The model under review builds one solid part; all positions refer to its coordinate system, in mm. Face numbers are marked on the shaded views. A direction names the side the tool comes from. Give positions to 0.01 mm unless a question says otherwise; leave off trailing zeros. Loops run counter-clockwise (first coordinate to the right, second up) from the corner with the lowest first, then second, coordinate; pieces in that order, holes last. Notation, with made-up numbers: (-2.75, 44) - (23.25, 44) arc R19 cw to (23.25, 50) - close; hole circle Ø8 at (26.5, -32.75). An arc over 180 degrees is marked (long way). Answer as a JSON object with one key per item and string values.
from build123d import *

# Parameters (mm, degrees)
ESQUISSE1_W        = 5
ESQUISSE1_H        = 5
BOSS_EXTRU_1_DEPTH = 5


with BuildPart() as part:
    # Esquisse1 → Boss.-Extru.1 (new body)
    with BuildSketch(Plane.XY):
        with BuildLine():
            Line((-62, 0), (-70, 0))
            Line((-70, 0), (-70, -5))
            Line((-70, -5), (-75, -5))
            Line((-75, -5), (-75, 0))
            Line((-75, 0), (-78.5, 0))
            Line((-78.5, 0), (-78.5, 3))
            Line((-78.5, 3), (-77.4, 3))
            Line((-77.4, 3), (-77.4, 5.3))
            Line((-77.4, 5.3), (-78.5, 5.3))
            Line((-78.5, 5.3), (-78.5, 10))
            Line((-78.5, 10), (-81.5, 10))
            Line((-81.5, 10), (-81.5, 5.3))
            Line((-81.5, 5.3), (-82.6, 5.3))
            Line((-82.6, 5.3), (-82.6, 3))
            Line((-82.6, 3), (-81.5, 3))
            Line((-81.5, 3), (-81.5, 0))
            Line((-81.5, 0), (-85, 0))
            Line((-85, 0), (-85, -5))
            Line((-85, -5), (-90, -5))
            Line((-90, -5), (-90, 0))
            Line((-90, 0), (-98, 0))
            ThreePointArc((-98, 0), (-99.414213562, 0.585786438), (-100, 2))
            Line((-100, 2), (-100, 10))
            Line((-100, 10), (-97.222166499, 42.643036354))
            ThreePointArc((-97.222166499, 42.643036354), (-89.672333618, 59.342381794), (-73.306153302, 67.589578681))
            ThreePointArc((-73.306153302, 67.589578681), (-70.002900284, 68.614551275), (-67.24637377, 70.70347705))
            ThreePointArc((-67.24637377, 70.70347705), (-37.614790527, 91.960082654), (-2.044554135, 99.999503671))
            ThreePointArc((-2.044554135, 99.999503671), (-0.601627423, 99.429879063), (0, 98))
            Line((0, 98), (0, 90))
            Line((0, 90), (5, 90))
            Line((5, 90), (5, 85))
            Line((5, 85), (0, 85))
            Line((0, 85), (0, 81.5))
            Line((0, 81.5), (-3, 81.5))
            Line((-3, 81.5), (-3, 82.6))
            Line((-3, 82.6), (-5.3, 82.6))
            Line((-5.3, 82.6), (-5.3, 81.5))
            Line((-5.3, 81.5), (-10, 81.5))
            Line((-10, 81.5), (-10, 78.5))
            Line((-10, 78.5), (-5.3, 78.5))
            Line((-5.3, 78.5), (-5.3, 77.4))
            Line((-5.3, 77.4), (-3, 77.4))
            Line((-3, 77.4), (-3, 78.5))
            Line((-3, 78.5), (0, 78.5))
            Line((0, 78.5), (0, 75))
            Line((0, 75), (5, 75))
            Line((5, 75), (5, 70))
            Line((5, 70), (0, 70))
            Line((0, 70), (0, 62))
            ThreePointArc((0, 62), (-0.585786438, 60.585786438), (-2, 60))
            Line((-2, 60), (-33.594430088, 60))
            ThreePointArc((-33.594430088, 60), (-41.52653458, 56.08947603), (-43.254902123, 47.416343664))
            ThreePointArc((-43.254902123, 47.416343664), (-42.980213788, 46.295555399), (-42.752787596, 45.164229918))
            ThreePointArc((-42.752787596, 45.164229918), (-43.187469445, 43.527910846), (-44.721399423, 42.811288741))
            Line((-44.721399423, 42.811288741), (-51.993903733, 42.811288741))
            ThreePointArc((-51.993903733, 42.811288741), (-55.195960034, 43.737154782), (-57.409791273, 46.22901026))
            ThreePointArc((-57.409791273, 46.22901026), (-83.571200219, 40.311288741), (-57.409791273, 34.393567223))
            ThreePointArc((-57.409791273, 34.393567223), (-55.195960034, 36.885422701), (-51.993903733, 37.811288741))
            Line((-51.993903733, 37.811288741), (-44.721399423, 37.811288741))
            ThreePointArc((-44.721399423, 37.811288741), (-43.187469445, 37.094666637), (-42.752787596, 35.458347565))
            ThreePointArc((-42.752787596, 35.458347565), (-47.057034679, 24.882654088), (-55.285653392, 16.96674166))
            ThreePointArc((-55.285653392, 16.96674166), (-58.742326175, 13.332888367), (-60, 8.477815449))
            Line((-60, 8.477815449), (-60, 2))
            ThreePointArc((-60, 2), (-60.585786438, 0.585786438), (-62, 0))
        make_face()
        with Locations((-69.821200219, 60.711288741)):
            Rectangle(ESQUISSE1_W, ESQUISSE1_H, mode=Mode.SUBTRACT)
        Polygon((-51.239218472, 53.926352251), (-48.739218472, 49.596225232), (-53.069345491, 47.096225232), (-55.569345491, 51.426352251), align=None, mode=Mode.SUBTRACT)
        Polygon((-48.739218472, 31.026352251), (-51.239218472, 26.696225232), (-55.569345491, 29.196225232), (-53.069345491, 33.526352251), align=None, mode=Mode.SUBTRACT)
        with Locations((-69.821200219, 19.911288741)):
            Rectangle(ESQUISSE1_W, ESQUISSE1_H, mode=Mode.SUBTRACT)
        Polygon((-88.403181966, 26.696225232), (-90.903181966, 31.026352251), (-86.573054947, 33.526352251), (-84.073054947, 29.196225232), align=None, mode=Mode.SUBTRACT)
        Polygon((-90.903181966, 49.596225232), (-88.403181966, 53.926352251), (-84.073054947, 51.426352251), (-86.573054947, 47.096225232), align=None, mode=Mode.SUBTRACT)
    extrude(amount=BOSS_EXTRU_1_DEPTH)


solid = part.part
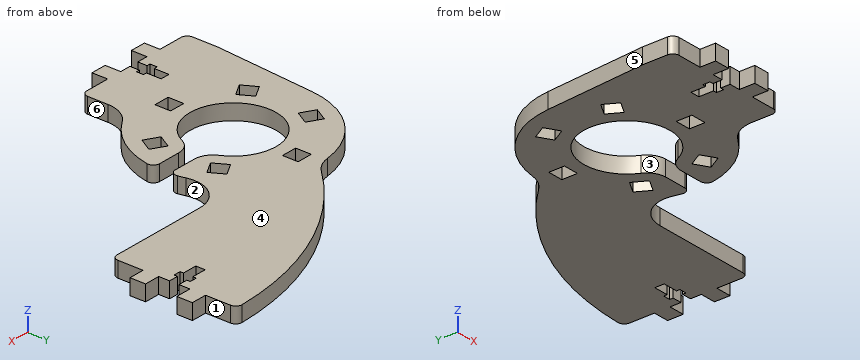
Q1. The part is to be moulded in two halves that separate along X. For the marked faces 3, 4, 5 and 6, say which applies: +X half, -X half, draft (parallel to the pull), parting line (faces both ways), or undercut.
Results:
{"face 3": "undercut", "face 4": "draft", "face 5": "-X half", "face 6": "+X half"}
Q2. For the marked faces 1 and 2, list the 3-axis set-ups (+Z, -Z, +X, -X, +Y, -Y) from which the entire face can be reached by the end or side of a thin tool; tool diameter is ignored.
Results:
{"face 1": "+Z, -Z, +X, +Y", "face 2": "+Z, -Z, +X"}
Q3. To check wall thickness, follow probe 1 along Y at (x, z) = (-52, 0.75); probe 2 along Y at (x, z) = (-88, 2.45); probe 3 along Y at (x, z) = (-71.5, 3.8). State the ranges of each line that lie inside material, in increasing order. Write a range as [from, to].
Results:
{"probe 1": "y = [19.37, 27.14], [32.91, 37.81], [42.81, 47.71], [53.49, 83.87]", "probe 2": "y = [-5, 26.93], [32.7, 47.92], [53.69, 60.95]", "probe 3": "y = [-5, 17.41], [22.41, 26.66], [53.96, 58.21], [63.21, 67.99]"}
Q4. Consider section A-A, the plane z = 2.55. State how many separate pieces and enclosed holes the cut face has, plus the area to 3 significant figures.
Results:
{"separate pieces": "1", "enclosed holes": "6", "area": "4,360 mm^2"}
Q5. Clearance check with flat-ended pins moving along their axes: pin 1 Ø0.9 at (y, z) = (78, 1.5) entering from -X; pin 2 Ø2 at (x, z) = (-58, 1) entering from +Y; pin 3 Ø4 at (x, y) = (-80.5, 32.5) entering from -Z; pin 4 Ø1.5 at (x, z) = (-70, 2) entering from +Y. State where each tip first meets the part, or that it passes through.
Results:
{"pin 1": "stops at x = -60.17", "pin 2": "stops at y = 80.18", "pin 3": "stops at z = 0", "pin 4": "stops at y = 69.04"}
Q6. Consider section B-B, the plane x = -14. State the section outline as (y, z) points, plus the area to 3 significant figures.
Results:
{"outline": "(60, 0) - (98.95, 0) - (98.95, 5) - (60, 5) - close", "area": "195 mm^2"}
